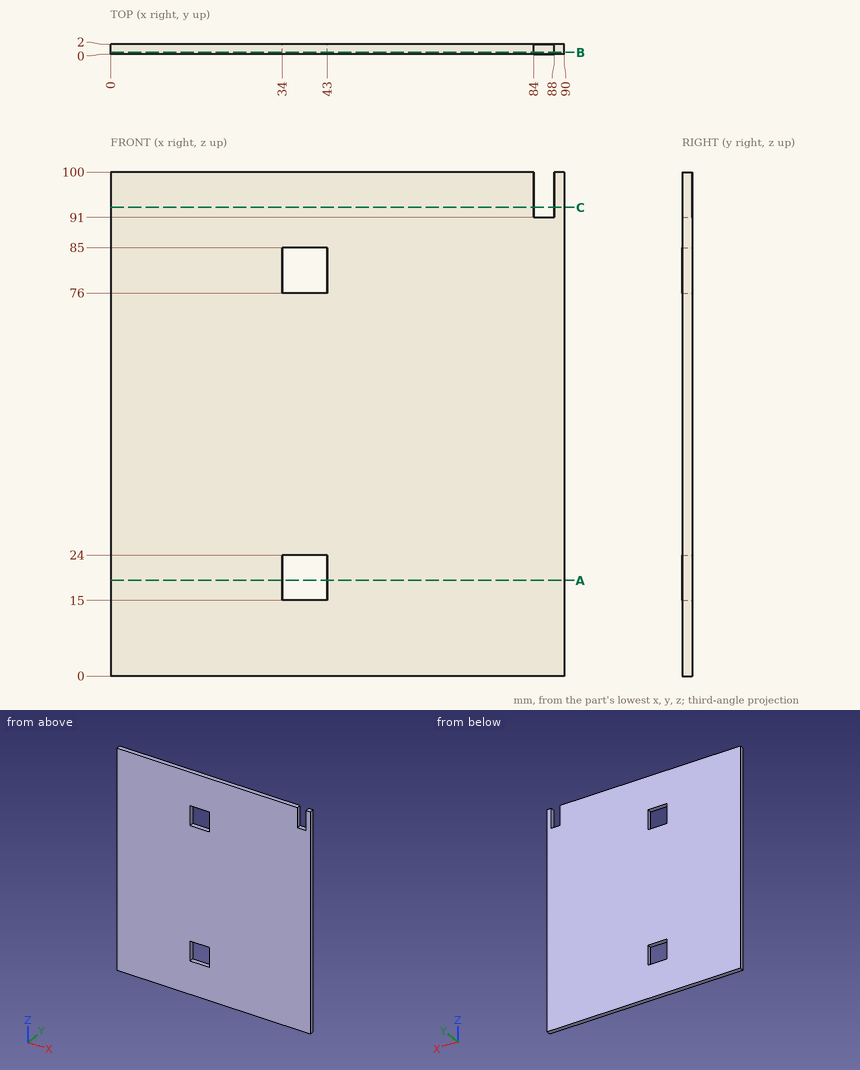
Check sheet for the drawn part. Datum: minimum x, y, z corner. Units: mm. Round coordinates to 2 decimals unless told otherwise and drop trailing zeros. Loops run counter-clockwise (first coordinate to the right, second up) from the corner with the lowest first, then second, coordinate; pieces in that order, holes last. Notation, with made-up numbers: M 69,64 L 120,64 A26 ccw 120,88 Z; hole C 23.25,71 d11. An arc over 180 degrees is marked long. Write each question's results on one line, items separated by ' | '.
1) Section check A-A on z = 19. Record the boundary of the cut face in (x, y), then the cut area to 3 significant figures.
Checks:
outline: M 0,0 L 34,0 L 34,2 L 0,2 Z; M 43,0 L 90,0 L 90,2 L 43,2 Z | area: 162 mm2
2) Section check C-C on z = 93. Record the boundary of the cut face in (x, y), then the cut area to 3 significant figures.
Checks:
outline: M 0,0 L 84,0 L 84,2 L 0,2 Z; M 88,0 L 90,0 L 90,2 L 88,2 Z | area: 172 mm2
3) Scan lines: L1, parallel to Z at x = 38.5, y = 0.85; L2, parallel to X at y = 1.05, z = 92; L3, parallel to X at y = 1.45, z = 15.5. Record each from-to range of solid material in increasing order. Write a range as from..to.
Checks:
L1: z = 0..15, 24..76, 85..100 | L2: x = 0..84, 88..90 | L3: x = 0..34, 43..90
4) Section check B-B on y = 0.35. Record the boundary of the cut face in (x, z).
Checks:
outline: M 0,0 L 90,0 L 90,100 L 88,100 L 88,91 L 84,91 L 84,100 L 0,100 Z; hole M 34,15 L 43,15 L 43,24 L 34,24 Z; hole M 34,76 L 43,76 L 43,85 L 34,85 Z
